Autodesk Inventor part; units mm, degrees
ref_plane "YZ Plane" through (0, 0, 0) normal (1, 0, 0) x (0, 1, 0)
ref_plane "XZ Plane" through (0, 0, 0) normal (0, 1, 0) x (-1, 0, 0)
ref_plane "XY Plane" through (0, 0, 0) normal (0, 0, 1) x (1, 0, 0)
sketch "草圖1" plane through (0, 0, 0) normal (0, 0, 1) x (1, 0, 0)
  line L0 (0, 0) -> (50, 0)
  line L1 (50, 0) -> (50, 20)
  line L2 (50, 20) -> (30, 40)
  line L3 (30, 40) -> (0, 40)
  line L4 (0, 40) -> (0, 0)
  dimension "d0" = 40
  dimension "d1" = 50
  dimension "d2" = 20
  dimension "d3" = 30
extrude "擠出1" add sketch "草圖1" along normal blind 10
sketch "草圖2" plane through (0, 0, 10) normal (0, 0, 1) x (1, 0, 0)
  line L0 (30, 40) -> (0, 40)
  line L1 (0, 40) -> (0, 0)
  line L2 (50, 0) -> (50, 20)
  line L3 (0, 0) -> (50, 0)
  line L4 (50, 0) -> (50, 10)
  line L5 (50, 10) -> (40, 10)
  line L6 (40, 10) -> (40, 20)
  line L7 (40, 20) -> (20, 20)
  line L8 (20, 20) -> (20, 30)
  line L9 (20, 30) -> (10, 30)
  line L10 (10, 30) -> (10, 40)
  line L11 (10, 40) -> (0, 40)
  dimension "d6" = 10
  dimension "d7" = 10
  dimension "d8" = 10
  dimension "d9" = 10
  dimension "d10" = 20
extrude "擠出2" add sketch "草圖2" along normal blind 30
chamfer "倒角1" distance 10 distance2 30 1 edges at (40, 15, 40) measured on face at (20, 10, 40)
Input: part model. Units: mm. Frame: model coordinates. A direction names the side the tool comes from. Round coordinates to 2 decimals unless told otherwise and drop trailing zeros. Loops run counter-clockwise (first coordinate to the right, second up) from the corner with the lowest first, then second, coordinate; pieces in that order, holes last.
1) Section query D-D on y = 37.5. Return the cut outline in (x, z), plus the area to 3 significant figures.
Ans:
outline: (0, 0) - (32.5, 0) - (32.5, 10) - (10, 10) - (10, 40) - (0, 40) - close
area: 625 mm2
2) Set-up query: faces 1 (the flat face through (20, 25, 25)), 2 (the flat face through (25, 0, 20)). Return all of +Z, -Z, +X, -X, +Y, -Y with unobstructed straight access to the full face (end or side cutting, diameter ignored); none if empty.
Ans:
face 1: +Z, +X, +Y
face 2: +Z, -Z, +X, -X, -Y
3) Pin query (flat end, axial travel): pin 1 (10 mm diameter, centred on x = 30.5, z = 21, fed in from +Y); pin 2 (6 mm diameter, centred on x = 40, z = 23.5, fed in from +Y); pin 3 (3 mm diameter, centred on y = 37, z = 27, fed in from +X). Return the tip coordinate at first contact, or that it passes through.
Ans:
pin 1: stops at y = 20
pin 2: stops at y = 10
pin 3: stops at x = 10
4) Section query C-C on x = 31. Return the cut outline in (y, z).
Ans:
outline: (0, 0) - (39, 0) - (39, 10) - (20, 10) - (20, 37) - (10, 37) - (10, 40) - (0, 40) - close
5) Material intervals for line 1 (Y direction, x = 33.5, z = 34); line 2 (Y direction, x = 15.5, z = 23); line 3 (X direction, y = 30, z = 6), sorted ascending.
Ans:
line 1: y = 0 to 10
line 2: y = 0 to 30
line 3: x = 0 to 40
6) Section query B-B on z = 3. Return the cut outline in (x, y), plus the area to 3 significant figures.
Ans:
outline: (0, 0) - (50, 0) - (50, 20) - (30, 40) - (0, 40) - close
area: 1,800 mm2
